```python
from build123d import *

# Parameters (mm, degrees)
F0_R     = 3.5
F1_DEPTH = 3
F2_R     = 7.5
F2_R_2   = 3.5
F3_DEPTH = 15
F4_R     = 2.5
F5_DEPTH = 3
F6_R     = 2.5
F7_DEPTH = 10
F8_R     = 4
F9_R     = 2


with BuildPart() as f1:
    # F0 (on Top) → F1 (new body)
    with BuildSketch(Plane.XY):
        Circle(F0_R)
    extrude(amount=F1_DEPTH)

    # F2 (on face) → F3 (join)
    with BuildSketch(Plane.XY.offset(3)):
        Circle(F2_R)
        Circle(F2_R_2, mode=Mode.SUBTRACT)
        Circle(F2_R_2)
    extrude(amount=F3_DEPTH)

    # F4 (on face) → F5 (join)
    with BuildSketch(Plane.XY.offset(18)):
        Circle(F4_R)
    extrude(amount=F5_DEPTH)

    # F6 (on face) → F7 (cut)
    with BuildSketch(Plane(origin=(0, 0, 0), x_dir=(1, 0, 0), z_dir=(0, 0, -1))):
        Circle(F6_R)
    extrude(amount=-F7_DEPTH, mode=Mode.SUBTRACT)

    # F8
    f8_edges = [f1.edges().sort_by_distance(p)[0] for p in [
        (-7.5, 0, 18),
    ]]
    fillet(f8_edges, radius=F8_R)

    # F9
    f9_edges = [f1.edges().sort_by_distance(p)[0] for p in [
        (-7.5, 0, 3),
    ]]
    fillet(f9_edges, radius=F9_R)


solid = f1.part
```
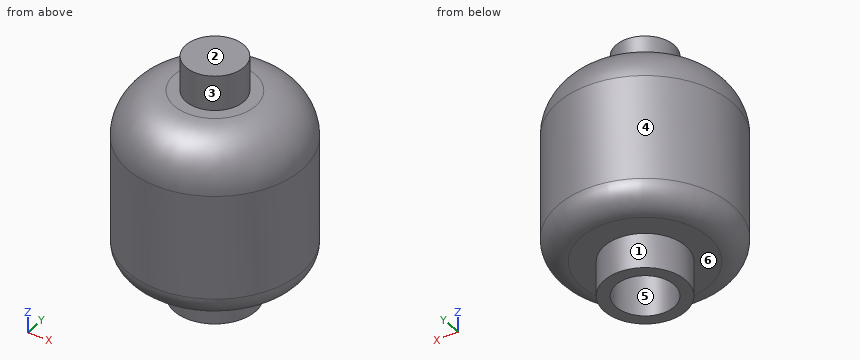
CAD build for the part. Positions are in the model's coordinates, mm. Face numbers are marked on the shaded views. A direction names the side the tool comes from. Give positions to 0.01 mm unless a question says otherwise; leave off trailing zeros. Write each loop counter-clockwise with the first axis right and the second up, starting at its lowest first coordinate (ties: lowest second). Pieces come first, ordered by that corner, then holes. Notation, with made-up numbers: M -37,74 L -7,74 A21 cw -7,111 Z; hole C 7,45.25 d1. An arc over 180 degrees is marked long. Return JSON: item names as keys, results as strings. Group by question number.
(1) Band-saw the part on B-B (z = 13.75). Give the cut face in (x, y).
(2) Mould opens along Y. For the marked faces 4, 5 and 6 say: pulls with the +Y half, pulls with the -Y half, needs draft (parallel to the pull), parting line crosses it, or undercut.
(3) Band-saw the part on A-A (z = 2.25). Give the cut face in (x, y).
(4) Flat gauge pins, fed straight in: pin 1 Ø6 at (y, z) = (-5, 8) entering from +X; pin 2 Ø3 at (y, z) = (3, 17.5) entering from -X; pin 3 Ø5 at (x, z) = (-4.5, 13) entering from -Y. Where does each tip first touch, or does it go through?
(5) 3-axis set-ups, long thin cutter, end or side, ignore diameter. For the marked faces 1, 2 and 3: which of +Z, -Z, +X, -X, +Y, -Y reach the whole face in a straight line?
(6) Band-saw the part on C-C (z = 9.75). Give the cut face in (x, y), and give its area (3 significant figures).
(7) Drill centre lines: L1, parallel to Y at x = 0, z = 5.25; L2, parallel to Z at x = -3.5, y = -1; L3, parallel to Z at x = -1.5, y = 1.75. Where is each one in solid material? Low to high. Write a range as [from, to].
Entries:
{
 "1": {"outline": "C 0,0 d15"},
 "2": {"face 4": "parting line crosses it", "face 5": "undercut", "face 6": "needs draft"},
 "3": {"outline": "C 0,0 d7; hole C 0,0 d5"},
 "4": {"pin 1": "stops at x = 7.23", "pin 2": "stops at x = -6.46", "pin 3": "stops at y = -7.23"},
 "5": {"face 1": "-Z", "face 2": "+Z, +X, -X, +Y, -Y", "face 3": "+Z"},
 "6": {"outline": "C 0,0 d15; hole C 0,0 d5", "area": "157 mm^2"},
 "7": {"L1": "y = [-7.5, -2.5], [2.5, 7.5]", "L2": "z = [3, 18]", "L3": "z = [10, 21]"}
}
